Check sheet for the modelled part. Datum: model origin and axes. Units: mm. Face numbers are marked on the shaded views. A direction names the side the tool comes from. Coordinates: 2 decimals unless noted, no trailing zeros. Loops run counter-clockwise (first coordinate to the right, second up) from the corner with the lowest first, then second, coordinate; pieces in that order, holes last. Notation, with made-up numbers: (22, 12.25) - (31, 12.25) arc R25 ccw to (31, 40.25) - close; hole circle Ø5 at (51.5, -27). An arc over 180 degrees is marked (long way). Write each question's results on one line, items separated by ' | '. Start each with the question number.
1. Cross-section at B-B (x = 0). Record the cut outline in (y, z), and give its area (3 significant figures).
2. Cross-section at D-D (y = -4.75). Record the cut outline in (x, z).
3. Cross-section at C-C (y = -1.5). Record the cut outline in (x, z).
4. Gauge pin test, flat ends, axial feed: P1, Ø1, axis at y = -7, z = -13.5, coming from the -X side; P2, Ø2, axis at y = -9, z = -10, coming from the -X side; P3, Ø2, axis at x = 9, z = -11.5, coming from the -Y side. Record the tip position at first contact, or that the pin passes through.
5. Thickness scan on line 1 (X direction, y = -6.3, z = 0); line 2 (X direction, y = -9.95, z = 0); line 3 (Y direction, x = 10.5, z = 9). Record the ranges inside material, lowest first. Write a range as [from, to].
6. Draft check along X on the marked faces 3, 4, 5 and 6. Enter one of: released by +X, released by -X, zero draft, split by the parting line, or undercut.
7. Cross-section at A-A (z = 0). Record the cut outline in (x, y), and give its area (3 significant figures).
8. Tool access check on the marked faces 1 and 2. Record the directions out of +Z, -Z, +X, -X, +Y, -Y that give a thin tool (end or side, any length) a straight path to the whole face; none if there is none.
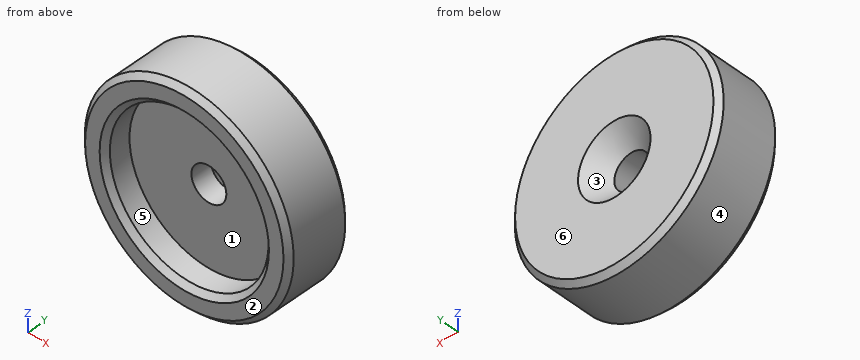
Autodesk Inventor part; units mm, degrees
ref_plane "YZ Plane" through (0, 0, 0) normal (1, 0, 0) x (0, 1, 0)
ref_plane "XZ Plane" through (0, 0, 0) normal (0, 1, 0) x (-1, 0, 0)
ref_plane "XY Plane" through (0, 0, 0) normal (0, 0, 1) x (1, 0, 0)
sketch "Skizze1" plane through (0, 0, 0) normal (1, 0, 0) x (0, 1, 0)
  line L0 (-15, 0) -> (2.5, 0)
  line L1 (0, 23.7) -> (0, -3.95) construction
  line L2 (0, 0) -> (0, 19.75)
  line L3 (0, 19.75) -> (-12.5, 19.75)
  line L4 (-12.5, 19.75) -> (-12.5, 15)
  line L5 (-12.5, 15) -> (-7.5, 15)
  line L6 (-7.5, 15) -> (-7.5, 0)
  line L7 (0, 0) -> (-7.5, 0)
  dimension "d0" = 12.5
  dimension "d1" = 39.5
  dimension "d2" = 30
  dimension "d3" = 5
revolve "Grundkoerper" add sketch "Skizze1" angle 360 about axis through (0, 0, 0) along (0, 1, 0)
sketch "Skizze2" plane through (0, 0, 0) normal (0, 1, 0) x (1, 0, 0)
  line L0 (0, 27.65) -> (0, -27.65) construction
  line L1 (27.65, 0) -> (-27.65, 0) construction
  point P0 (0, 0)
  point P1 (0, 0)
hole "BOH_M6_ISO10642" at (0, 0, 0) direction (0, -1, 0) diameter 6.6 end through all countersink diameter 13.7 countersink angle 90
chamfer "Fase1" distance 1 angle 45 3 edges at (0, -12.5, -15) (0, -12.5, -19.75) (0, 0, -19.75)
properties part number "200-20-ROCKER-CONNECTOR-02" material "Aluminium 6061"
Established:
1) outline: (-12.5, -18.75) - (-11.5, -19.75) - (-1, -19.75) - (0, -18.75) - (0, -6.85) - (-3.55, -3.3) - (-7.5, -3.3) - (-7.5, -15) - (-11.5, -15) - (-12.5, -16) - close; (-12.5, 16) - (-11.5, 15) - (-7.5, 15) - (-7.5, 3.3) - (-3.55, 3.3) - (0, 6.85) - (0, 18.75) - (-1, 19.75) - (-11.5, 19.75) - (-12.5, 18.75) - close | area: 279 mm^2
2) outline: circle Ø39.5 at (0, 0); hole circle Ø6.6 at (0, 0)
3) outline: circle Ø39.5 at (0, 0); hole circle Ø10.7 at (0, 0)
4) P1: x = -14.87 | P2: x = -17.58 | P3: y = -12.1
5) line 1: [-19.75, -3.3], [3.3, 19.75] | line 2: [-19.75, -15], [15, 19.75] | line 3: [-7.5, 0]
6) face 3: undercut | face 4: split by the parting line | face 5: undercut | face 6: zero draft
7) outline: (-19.75, -11.5) - (-18.75, -12.5) - (-16, -12.5) - (-15, -11.5) - (-15, -7.5) - (-3.3, -7.5) - (-3.3, -3.55) - (-6.85, 0) - (-18.75, 0) - (-19.75, -1) - close; (3.3, -7.5) - (15, -7.5) - (15, -11.5) - (16, -12.5) - (18.75, -12.5) - (19.75, -11.5) - (19.75, -1) - (18.75, 0) - (6.85, 0) - (3.3, -3.55) - close | area: 279 mm^2
8) face 1: -Y | face 2: +Z, -Z, +X, -X, -Y
